Input: part model. Units: mm. Frame: model coordinates. A direction names the side the tool comes from. Give positions to 0.01 mm unless a question says otherwise; leave off trailing zeros. Order: outer loops, then holes, each group sorted by start corner. A loop starts at its lowest first (then second) coordinate and runs counter-clockwise, first axis right, second up. Notation, with made-up numbers: (88.5, 89.5) - (129.5, 89.5) arc R20 cw to (129.5, 122.5) - close; hole circle Ø6 at (-19, -29.5). An arc over 180 degrees is marked (long way). Answer in a Markdown table with one row per item. Add a question column.
1. Section query B-B on x = 41.5. Return loops of the section in (y, z).
2. Section query C-C on x = 37.75. Return loops of the section in (y, z), and give its area (3 significant figures).
3. Section query D-D on y = 43. Return loops of the section in (x, z).
4. Mould query, pull axis Z, two halves, no side actions, for faces 1 (the face through (47.479, 12.368, 9.976)), 2 (the face through (41, 28, 7)), 3 (the face through (47.52, -13.14, 19.1)). Classes: released by +Z, released by -Z, zero draft, split by the parting line, or undercut.
5. Contact query for flat-ended pins moving along their axis: pin 1 (3 mm diameter, centred on x = 40.5, z = 13.5, fed in from +Y); pin 2 (3 mm diameter, centred on x = 38.5, y = 31, fed in from -Z); pin 3 (8 mm diameter, centred on y = 13.5, z = 26.5, fed in from -X); pin 4 (0.9 mm diameter, centred on x = 47.5, y = 1, fed in from +Z). Output: stop coordinate, or through.
6. Ray query, line 1 (Y direction, x = 47.1, z = 11.5); line 2 (X direction, y = 43, z = 29.75); line 3 (Y direction, x = 41.5, z = 32.2). Return the intervals inside material, ascending. Write a range as [from, to].
7. Section query A-A on y = 13. Return loops of the section in (x, z), and give its area (3 significant figures).
8. Access query for faces 4 (the face through (47, 2, 20)), 5 (the face through (41, 34, 29)), 6 (the face through (41, 49, 29)), 7 (the face through (41, 30, 15.9)). Directions: +Z, -Z, +X, -X, +Y, -Y. A direction counts if a zero-diameter tool reaches every point of the face in a straight line with its end or side. Return the directions, or none.
```python
from build123d import *

# Parameters (mm, degrees)
BOX055_W           = 15
BOX055_H           = 2
BOX055_DEPTH       = 26
FILLET005015025_R  = 3
BOX058_W           = 15
BOX058_H           = 6
BOX058_DEPTH       = 5.8
FILLET005015028_R  = 1
CYLINDER021_R      = 3.15
CYLINDER021_DEPTH  = 10
BOX054_W           = 15
BOX054_H           = 24.5
BOX054_DEPTH       = 5
CHAMFER010013_SIZE = 1
BOX057_W           = 15
BOX057_H           = 7.8
BOX057_DEPTH       = 2
CYLINDER023_R      = 1.65
CYLINDER023_DEPTH  = 14
CYLINDER022_R      = 1.65
CYLINDER022_DEPTH  = 14
BOX056_W           = 3
BOX056_H           = 40
BOX056_DEPTH       = 17
FILLET005015024_R  = 3
CHAMFER010014_SIZE = 12
CHAMFER010015_SIZE = 1


with BuildPart() as fillet005015025:
    # Box055 → Box055 (new body)
    with BuildSketch(Plane(origin=(34, 26, 3), x_dir=(1, 0, 0), z_dir=(0, 0, 1))):
        with Locations((7.5, 1)):
            Rectangle(BOX055_W, BOX055_H)
    extrude(amount=BOX055_DEPTH)

    # Fillet005015025
    fillet005015025_edges = [fillet005015025.edges().sort_by_distance(p)[0] for p in [
        (34, 27, 3),
    ]]
    fillet(fillet005015025_edges, radius=FILLET005015025_R)


with BuildPart() as fillet005015028:
    # Box058 → Box058 (new body)
    with BuildSketch(Plane(origin=(34, 27, 10.1), x_dir=(1, 0, 0), z_dir=(0, 0, 1))):
        with Locations((7.5, 3)):
            Rectangle(BOX058_W, BOX058_H)
    extrude(amount=BOX058_DEPTH)

    # Fillet005015028
    fillet005015028_edges = [fillet005015028.edges().sort_by_distance(p)[0] for p in [
        (41.5, 33, 10.1),
        (41.5, 33, 15.9),
    ]]
    fillet(fillet005015028_edges, radius=FILLET005015028_R)


with BuildPart() as cylinder021:
    # Cylinder021 → Cylinder021 (new body)
    with BuildSketch(Plane(origin=(41.5, 43, 25), x_dir=(1, 0, 0), z_dir=(0, 0, 1))):
        Circle(CYLINDER021_R)
    extrude(amount=CYLINDER021_DEPTH)


with BuildPart() as chamfer010013:
    # Box054 → Box054 (new body)
    with BuildSketch(Plane(origin=(34, 26, 29), x_dir=(1, 0, 0), z_dir=(0, 0, 1))):
        with Locations((7.5, 12.25)):
            Rectangle(BOX054_W, BOX054_H)
    extrude(amount=BOX054_DEPTH)

    # Chamfer010013
    chamfer010013_edges = [chamfer010013.edges().sort_by_distance(p)[0] for p in [
        (34, 50.5, 31.5),
        (49, 50.5, 31.5),
    ]]
    chamfer(chamfer010013_edges, length=CHAMFER010013_SIZE)


with BuildPart() as cut019003006:
    # Box057 → Box057 (new body)
    with BuildSketch(Plane(origin=(34, 39.1, 28), x_dir=(1, 0, 0), z_dir=(0, 0, 1))):
        with Locations((7.5, 3.9)):
            Rectangle(BOX057_W, BOX057_H)
    extrude(amount=BOX057_DEPTH)

    # Fusion001021004009015012: union Chamfer010013
    add(chamfer010013.part)

    # Cut019003006: cut Cylinder021
    add(cylinder021.part, mode=Mode.SUBTRACT)


with BuildPart() as cylinder023:
    # Cylinder023 → Cylinder023 (new body)
    with BuildSketch(Plane(origin=(37, 13, 11.5), x_dir=(0, 0, -1), z_dir=(1, 0, 0))):
        Circle(CYLINDER023_R)
    extrude(amount=CYLINDER023_DEPTH)


with BuildPart() as fusion001021004009015011:
    # Cylinder022 → Cylinder022 (new body)
    with BuildSketch(Plane(origin=(37, -6, 11.5), x_dir=(0, 0, -1), z_dir=(1, 0, 0))):
        Circle(CYLINDER022_R)
    extrude(amount=CYLINDER022_DEPTH)

    # Fusion001021004009015011: union Cylinder023
    add(cylinder023.part)


with BuildPart() as top_mount_arm_right:
    # Box056 → Box056 (new body)
    with BuildSketch(Plane(origin=(46, -14, 3), x_dir=(1, 0, 0), z_dir=(0, 0, 1))):
        with Locations((1.5, 20)):
            Rectangle(BOX056_W, BOX056_H)
    extrude(amount=BOX056_DEPTH)

    # Fillet005015024
    fillet005015024_edges = [top_mount_arm_right.edges().sort_by_distance(p)[0] for p in [
        (47.5, -14, 3),
        (47.5, -14, 20),
    ]]
    fillet(fillet005015024_edges, radius=FILLET005015024_R)

    # Cut019003007: cut Fusion001021004009015011
    add(fusion001021004009015011.part, mode=Mode.SUBTRACT)

    # Fusion001021004009015013: union Fillet005015025, Fillet005015028, Cut019003006
    add(fillet005015025.part)
    add(fillet005015028.part)
    add(cut019003006.part)

    # Chamfer010014
    chamfer010014_edges = [top_mount_arm_right.edges().sort_by_distance(p)[0] for p in [
        (47.5, 26, 20),
    ]]
    chamfer(chamfer010014_edges, length=CHAMFER010014_SIZE)

    # Chamfer010015
    chamfer010015_edges = [top_mount_arm_right.edges().sort_by_distance(p)[0] for p in [
        (41.5, 26, 34),
    ]]
    chamfer(chamfer010015_edges, length=CHAMFER010015_SIZE)


solid = top_mount_arm_right.part
```
Answer:
| question | item | result |
|---|---|---|
| 1 | outline | (26, 3) - (28, 3) - (28, 10.1) - (32, 10.1) arc R1 ccw to (33, 11.1) - (33, 14.9) arc R1 ccw to (32, 15.9) - (28, 15.9) - (28, 29) - (39.1, 29) - (39.1, 28) - (39.85, 28) - (39.85, 34) - (27, 34) - (26, 33) - close; (46.15, 28) - (46.9, 28) - (46.9, 29) - (50.5, 29) - (50.5, 34) - (46.15, 34) - close |
| 2 | outline | (26, 3) - (28, 3) - (28, 10.1) - (32, 10.1) arc R1 ccw to (33, 11.1) - (33, 14.9) arc R1 ccw to (32, 15.9) - (28, 15.9) - (28, 29) - (39.1, 29) - (39.1, 28) - (46.9, 28) - (46.9, 29) - (50.5, 29) - (50.5, 34) - (27, 34) - (26, 33) - close |
| 2 | area | 210 mm² |
| 3 | outline | (34, 28) - (38.35, 28) - (38.35, 34) - (34, 34) - close; (44.65, 28) - (49, 28) - (49, 34) - (44.65, 34) - close |
| 4 | face 1 | undercut |
| 4 | face 2 | zero draft |
| 4 | face 3 | released by +Z |
| 5 | pin 1 | stops at y = 33 |
| 5 | pin 2 | stops at z = 10.1 |
| 5 | pin 3 | passes through |
| 5 | pin 4 | stops at z = 20 |
| 6 | line 1 | y = [-14, -7.65], [-4.35, 11.35], [14.65, 33] |
| 6 | line 2 | x = [34, 38.35], [44.65, 49] |
| 6 | line 3 | y = [26, 39.85], [46.15, 50.5] |
| 7 | outline | (46, 3) - (49, 3) - (49, 9.85) - (46, 9.85) - close; (46, 13.15) - (49, 13.15) - (49, 20) - (46, 20) - close |
| 7 | area | 41.1 mm² |
| 8 | face 4 | +Z, +X, -X, -Y |
| 8 | face 5 | +X, -X |
| 8 | face 6 | -Z, +X, -X, +Y |
| 8 | face 7 | +X, -X, +Y |
